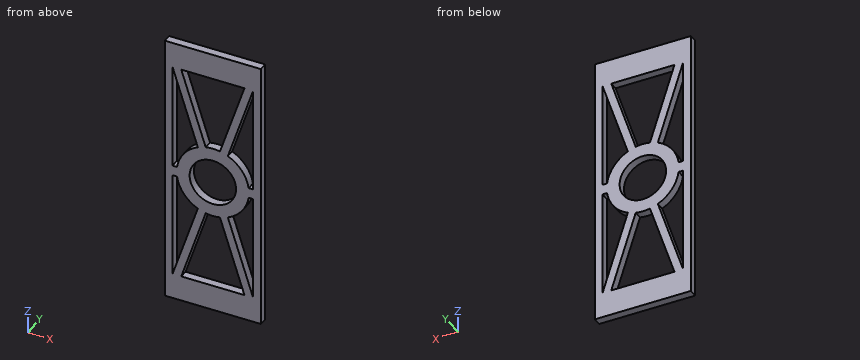
Autodesk Inventor part; units mm, degrees
ref_plane "YZ Plane" through (0, 0, 0) normal (1, 0, 0) x (0, 1, 0)
ref_plane "XZ Plane" through (0, 0, 0) normal (0, 1, 0) x (-1, 0, 0)
ref_plane "XY Plane" through (0, 0, 0) normal (0, 0, 1) x (1, 0, 0)
sketch "Sketch1" plane through (0, 0, 0) normal (0, 1, 0) x (-1, 0, 0)
  line L0 (15.3, 271) -> (-170.7, 271)
  line L1 (-170.7, 271) -> (-170.7, -271)
  line L2 (-170.7, -271) -> (15.3, -271)
  line L3 (15.3, -271) -> (15.3, 271)
  line L4 (-77.7, 271) -> (-77.7, -271)
  line L5 (-170.7, 0) -> (15.3, 0)
  circle A0 centre (-77.7, 0) radius 45
  point P0 (0, 0)
  dimension "d0" = 542
  dimension "d1" = 186
  dimension "d2" = 90
extrude "Extrusion1" add sketch "Sketch1" along normal blind 16 contours L3 L5 A0 L4 L0 | L4 A0 L5 L1 L0 | L3 L2 L4 A0 L5 | L5 A0 L4 L2 L1
sketch "Sketch2" plane through (170.7, 0, 271) normal (1, 0, 0) x (0, 0, -1)
  line L0 (0, 0) -> (0, 16)
  line L1 (0, 6) -> (-25, 6)
  line L2 (-25, 6) -> (-25, 0)
  line L3 (-25, 0) -> (0, 0)
  line L4 (0, 0) -> (0, 6)
  line L5 (542, 0) -> (542, 16)
  line L6 (542, 6) -> (567, 6)
  line L7 (567, 6) -> (567, 0)
  line L8 (567, 0) -> (542, 0)
  line L9 (542, 0) -> (542, 6)
  line L10 (542, 16) -> (527, 16)
  line L11 (527, 16) -> (527, 66)
  line L12 (527, 66) -> (542, 66)
  line L13 (542, 66) -> (542, 16)
  line L14 (0, 16) -> (15, 16)
  line L15 (15, 16) -> (15, 66)
  line L16 (15, 66) -> (0, 66)
  line L17 (0, 66) -> (0, 16)
  point P0 (271, 0)
  dimension "d5" = 6
  dimension "d6" = 25
  dimension "d7" = 25
  dimension "d8" = 50
  dimension "d9" = 15
  dimension "d10" = 15
  dimension "d11" = 50
extrude "Extrusion2" add sketch "Sketch2" against normal up to surface (186 mm away)
sketch "Sketch3" plane through (0, 16, 0) normal (0, 1, 0) x (1, 0, 0)
  line L0 (170.7, 256) -> (-15.3, 256)
  line L1 (-15.3, 256) -> (-15.3, -256)
  line L2 (-15.3, -256) -> (170.7, -256)
  line L3 (170.7, -256) -> (170.7, 256)
  circle A0 centre (77.7, 0) radius 45
  line L4 (-0.3, -241) -> (-0.3, 241)
  line L5 (-0.3, 241) -> (155.7, 241)
  line L6 (155.7, 241) -> (155.7, -241)
  line L7 (155.7, -241) -> (-0.3, -241)
  circle A1 centre (77.7, 0) radius 70
  line L8 (155.7, -241) -> (-0.3, 241)
  line L9 (155.7, 241) -> (-0.3, -241)
  line L10 (148.0887, 243.4634) -> (-7.9113, -238.5366)
  line L11 (163.3113, 238.5366) -> (7.3113, -243.4634)
  line L12 (148.0887, -243.4634) -> (-7.9113, 238.5366)
  line L13 (163.3113, -238.5366) -> (7.3113, 243.4634)
  line L14 (-0.3, -10) -> (155.7, -10)
  line L15 (155.7, -10) -> (155.7, 10)
  line L16 (155.7, 10) -> (-0.3, 10)
  line L17 (-0.3, 10) -> (-0.3, -10)
  point P0 (0, 0)
  point P1 (77.7, 0)
  point P2 (77.7, 0)
  point P3 (146.982, 10)
  point P4 (155.7, 215.0197)
  point P5 (106.7248, 63.699)
  point P6 (146.982, -10)
  point P7 (106.7248, -63.699)
  point P8 (155.7, -215.0197)
  point P9 (8.1086, 241)
  point P10 (63.8977, 68.6258)
  point P11 (91.5023, 68.6258)
  point P12 (147.2914, 241)
  point P13 (-0.3, 10)
  point P14 (8.418, 10)
  point P15 (48.6752, 63.699)
  point P16 (-0.3, 215.0197)
  point P17 (8.418, -10)
  point P18 (-0.3, -215.0197)
  point P19 (48.6752, -63.699)
  point P20 (147.2914, -241)
  point P21 (91.5023, -68.6258)
  point P22 (63.8977, -68.6258)
  point P23 (8.1086, -241)
  dimension "d14" = 25
  dimension "d15" = 15
  dimension "d16" = 10
  dimension "d17" = 10
  dimension "d18" = 8
  dimension "d19" = 8
  dimension "d20" = 8
  dimension "d21" = 8
extrude "Extrusion3" cut sketch "Sketch3" against normal blind 20 contours A1 L11 L6 L16 | L14 L6 L13 A1 | A1 L13 L5 L10 | L12 L7 L11 A1 | A1 L16 L4 L12 | L10 L4 L14 A1
sketch "Sketch4" plane through (0, 16, 0) normal (0, 1, 0) x (1, 0, 0)
  line L0 (-0.3, 10) -> (-0.3, 215.0197)
  line L1 (-0.3, 215.0197) -> (156, 215.0197)
  line L2 (156, 215.0197) -> (156, 245)
  line L3 (156, 245) -> (-0.3, 245)
  line L4 (-0.3, 245) -> (-0.3, 215.0197)
  line L5 (-0.3, -215.0197) -> (48.6752, -63.699)
  line L6 (-0.3, -215.0197) -> (158, -215.0197)
  line L7 (158, -215.0197) -> (158, -245)
  line L8 (158, -245) -> (-0.3, -245)
  line L9 (-0.3, -245) -> (-0.3, -215.0197)
  point P0 (0, 0)
extrude "Extrusion4" add sketch "Sketch4" against normal up to surface (16 mm away)
sketch "Sketch5" plane through (0, 16, 0) normal (0, 1, 0) x (1, 0, 0)
  line L0 (-72, -376) -> (216, -376)
  line L1 (216, -376) -> (216, -255.0197)
  line L2 (216, -255.0197) -> (-72, -255.0197)
  line L3 (-72, -255.0197) -> (-72, -376)
  line L4 (-67, 399) -> (218, 399)
  line L5 (218, 399) -> (218, 255.0197)
  line L6 (218, 255.0197) -> (-67, 255.0197)
  line L7 (-67, 255.0197) -> (-67, 399)
  line L8 (16.5171, 215.0197) -> (138.8829, 215.0197)
  line L9 (138.8829, -215.0197) -> (16.5171, -215.0197)
  point P0 (0, 0)
  dimension "d26" = 40
  dimension "d27" = 40
extrude "Extrusion5" cut sketch "Sketch5" along normal mid plane 100
sketch "Sketch6" plane through (0, 16, 0) normal (0, 1, 0) x (1, 0, 0)
  line L0 (-15.3, 255.0197) -> (-15.3, -255.0197)
  line L1 (-15.3, 255.0197) -> (170.7, 255.0197)
  line L2 (170.7, 255.0197) -> (170.7, 265.0197)
  line L3 (170.7, 265.0197) -> (-15.3, 265.0197)
  line L4 (-15.3, 265.0197) -> (-15.3, 255.0197)
  line L5 (-15.3, -255.0197) -> (170.7, -255.0197)
  line L6 (170.7, -255.0197) -> (170.7, -265.0197)
  line L7 (170.7, -265.0197) -> (-15.3, -265.0197)
  line L8 (-15.3, -265.0197) -> (-15.3, -255.0197)
  line L9 (-15.3, -255.0197) -> (170.7, -255.0197)
  point P0 (0, 0)
  dimension "d30" = 10
  dimension "d31" = 0
  dimension "d32" = 10
extrude "Extrusion6" add sketch "Sketch6" against normal up to surface (16 mm away)
properties part number "A_AxisKrovatka" material "Aluminum 6061"
Build history of the part. All positions in model axes, mm. Give positions to 0.01 mm unless a question says otherwise; leave off trailing zeros. Order: outer loops, then holes, each group sorted by start corner. A loop starts at its lowest first (then second) coordinate and runs counter-clockwise, first axis right, second up. Notation, with made-up numbers: M 44,-37 L 70,-37 A14 ccw 70,-16 Z; hole C -34.75,-27.75 d9. An arc over 180 degrees is marked long. Use one line per item in the form item = value.
1) Saw through at C-C (x = 77.7). Give the cut face in (y, z).
Calculated:
outline = M 0,-265.02 L 16,-265.02 L 16,-215.02 L 0,-215.02 Z; M 0,-70 L 16,-70 L 16,-45 L 0,-45 Z; M 0,45 L 16,45 L 16,70 L 0,70 Z; M 0,215.02 L 16,215.02 L 16,265.02 L 0,265.02 Z
2) Probe probe 1 along Z at (x, y) = (77.5, 9.25); probe 2 along X at (y, z) = (8, 0); probe 3 along X at (y, z) = (12.25, -162.5). List the from-to ranges inside material, lowest first.
Calculated:
probe_1 = -265.02 to -215.02, -70 to -45, 45 to 70, 215.02 to 265.02
probe_2 = -15.3 to 32.7, 122.7 to 170.7
probe_3 = -15.3 to -0.3, 16.7 to 33.52, 121.88 to 138.7, 155.7 to 170.7
3) Saw through at A-A (z = -56). Give the cut face in (x, y), plus the area to 3 significant figures.
Calculated:
outline = M -15.3,0 L -0.3,0 L -0.3,16 L -15.3,16 Z; M 35.7,0 L 119.7,0 L 119.7,16 L 35.7,16 Z; M 155.7,0 L 170.7,0 L 170.7,16 L 155.7,16 Z
area = 1,820 mm2
4) Saw through at B-B (z = 0). Give the cut face in (x, y).
Calculated:
outline = M -15.3,0 L 32.7,0 L 32.7,16 L -15.3,16 Z; M 122.7,0 L 170.7,0 L 170.7,16 L 122.7,16 Z
5) Saw through at D-D (y = 7). State how many separate pieces and enclosed holes the cut face has, plus the area to 3 significant figures.
Calculated:
separate_pieces = 1
enclosed_holes = 7
area = 50,900 mm2
